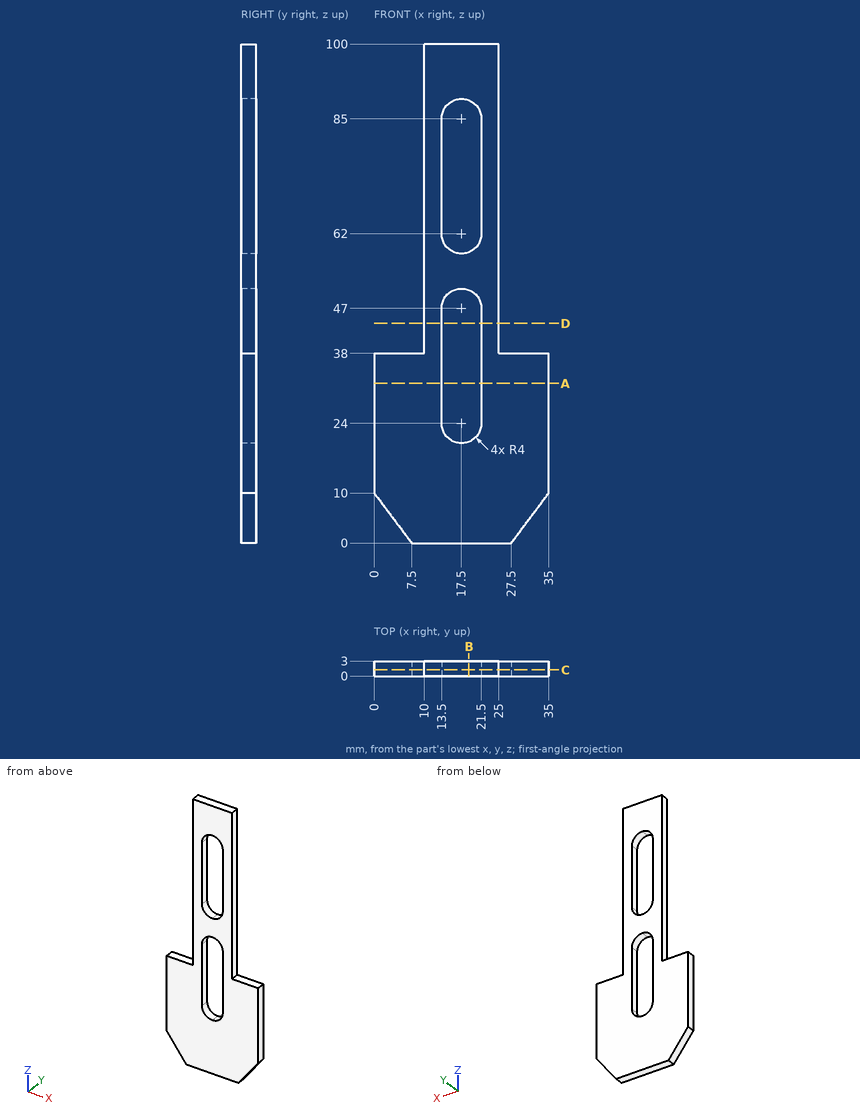
Here's the drawing with two shaded views (mm, measured from the low corner). I have some questions. Round coordinates to 2 decimals unless told otherwise and drop trailing zeros. Loops run counter-clockwise (first coordinate to the right, second up) from the corner with the lowest first, then second, coordinate; pieces in that order, holes last. Notation, with made-up numbers: (52.5, -40) - (103.5, -40) arc R34 cw to (103.5, -9) - close; hole circle Ø10 at (-34, -39). An arc over 180 degrees is marked (long way). Write item = value, one per line.
1) I need wall thicknesses on line 1 along X through (y, z) = (1.7, 72.5); line 2 along X through (y, z) = (0.3, 29.5); line 3 along X through (y, z) = (2.05, 52). Which ranges of each line are inside material? Lowest first, please. Write a range as from..to.
Computed:
line_1 = 10..13.5, 21.5..25
line_2 = 0..13.5, 21.5..35
line_3 = 10..25
2) Imagine slicing it at B-B (x = 19). Please give me the cut outline in (y, z), and give its area (3 significant figures).
Computed:
outline = (0, 0) - (3, 0) - (3, 20.29) - (0, 20.29) - close; (0, 50.71) - (3, 50.71) - (3, 58.29) - (0, 58.29) - close; (0, 88.71) - (3, 88.71) - (3, 100) - (0, 100) - close
area = 118 mm2
3) Imagine slicing it at C-C (y = 1.25). Please give me the cut outline in (x, z), and give its area (3 significant figures).
Computed:
outline = (0, 10) - (7.5, 0) - (27.5, 0) - (35, 10) - (35, 38) - (25, 38) - (25, 100) - (10, 100) - (10, 38) - (0, 38) - close; hole (13.5, 24) arc R4 ccw to (21.5, 24) - (21.5, 47) arc R4 ccw to (13.5, 47) - close; hole (13.5, 62) arc R4 ccw to (21.5, 62) - (21.5, 85) arc R4 ccw to (13.5, 85) - close
area = 1,720 mm2
4) Imagine slicing it at D-D (z = 44). Please give me the cut outline in (x, y), and give its area (3 significant figures).
Computed:
outline = (10, 0) - (13.5, 0) - (13.5, 3) - (10, 3) - close; (21.5, 0) - (25, 0) - (25, 3) - (21.5, 3) - close
area = 21.0 mm2
5) I'm going to push flat-ended pins straight in: P1, Ø10, axis at x = 26.5, z = 48.5, coming from the -Y side; P2, Ø1, axis at y = 1.5, z = 76.5, coming from the +X side; P3, Ø0.9, axis at x = 29.5, y = 2, coming from the +Z side. Where does each tip first touch, or does it pass through?
Computed:
P1 = 0
P2 = 25
P3 = 38
6) Imagine slicing it at A-A (z = 32). Please give me the cut outline in (x, y), and give its area (3 significant figures).
Computed:
outline = (0, 0) - (13.5, 0) - (13.5, 3) - (0, 3) - close; (21.5, 0) - (35, 0) - (35, 3) - (21.5, 3) - close
area = 81.0 mm2
